```python
from build123d import *

# Parameters (mm, degrees)
CROQUIS1_W              = 20
CROQUIS1_H              = 50
SALIENTE_EXTRUIR1_DEPTH = 3
CROQUIS2_W              = 20
CROQUIS2_H              = 3
SALIENTE_EXTRUIR2_DEPTH = 7
CROQUIS3_W              = 20
CROQUIS3_H              = 3
SALIENTE_EXTRUIR3_DEPTH = 7


with BuildPart() as part:
    # Croquis1 → Saliente-Extruir1 (new body)
    with BuildSketch(Plane.XY):
        Rectangle(CROQUIS1_W, CROQUIS1_H)
    extrude(amount=SALIENTE_EXTRUIR1_DEPTH)

    # Croquis2 → Saliente-Extruir2 (add)
    with BuildSketch(Plane(origin=(0, 0, 0), x_dir=(-1, 0, 0), z_dir=(0, 0, -1))):
        with Locations((0, 23.5)):
            Rectangle(CROQUIS2_W, CROQUIS2_H)
    extrude(amount=SALIENTE_EXTRUIR2_DEPTH)

    # Croquis3 → Saliente-Extruir3 (add)
    with BuildSketch(Plane(origin=(0, 0, 0), x_dir=(-1, 0, 0), z_dir=(0, 0, -1))):
        with Locations((0, -23.5)):
            Rectangle(CROQUIS3_W, CROQUIS3_H)
    extrude(amount=SALIENTE_EXTRUIR3_DEPTH)


solid = part.part
```
The listing builds one solid part. Answer for the finished solid, in the listing's coordinates (mm). A direction names the side the tool comes from. Coordinates: 2 decimals unless noted, no trailing zeros. Write each loop counter-clockwise with the first axis right and the second up, starting at its lowest first coordinate (ties: lowest second). Pieces come first, ordered by that corner, then holes. Notation, with made-up numbers: M 22,56 L 27,56 A13 cw 27,80 Z; hole C 1.25,-9.5 d5. An arc over 180 degrees is marked long. Use a Markdown table: item, result. Add a question column.
1. Section A-A (z = -2.75) is taken. Give the vertices of the cut face in (x, y).
2. For a pull along Y with two mould halves and no side action, classify faces 1 (the flat face through (0, 22, -3)), 2 (the flat face through (0, -25, -2)), 3 (the flat face through (0, -23, -7)) as +Y half, -Y half, draft (parallel to the pull), parting line (faces both ways), or undercut.
3. Section B-B (x = 4.5) is taken. Give the vertices of the cut face in (y, z).
4. Given P1, Ø8, axis at x = -0.5, y = -5.5, coming from the -Z side, flat-ended and moving along its own axis, determine where the tip first touches the part or whether it passes through.
5. Which of the six approach directions +Z, -Z, +X, -X, +Y, -Y give full straight-line access (tool end or side, diameter ignored) to faces 4 (the flat face through (0, 25, -2)), 5 (the flat face through (0, -22, -3))?
6. Straight lines are drawn through the part: line 1 along Y through (x, z) = (7.75, -5); line 2 along Z through (x, y) = (1.25, -4.5). For each, find the intervals that lie inside material, in ascending order. Write a range as [from, to].
7. Section C-C (y = 18) is taken. Give the vertices of the cut face in (x, z).
Data:
| question | item | result |
|---|---|---|
| 1 | outline | M -10,-25 L 10,-25 L 10,-22 L -10,-22 Z; M -10,22 L 10,22 L 10,25 L -10,25 Z |
| 2 | face 1 | undercut |
| 2 | face 2 | -Y half |
| 2 | face 3 | draft |
| 3 | outline | M -25,-7 L -22,-7 L -22,0 L 22,0 L 22,-7 L 25,-7 L 25,3 L -25,3 Z |
| 4 | P1 | stops at z = 0 |
| 5 | face 4 | +Z, -Z, +X, -X, +Y |
| 5 | face 5 | -Z, +X, -X |
| 6 | line 1 | y = [-25, -22], [22, 25] |
| 6 | line 2 | z = [0, 3] |
| 7 | outline | M -10,0 L 10,0 L 10,3 L -10,3 Z |
